```python
from build123d import *

# Parameters (mm, degrees)
SKETCH044_W             = 574.323184
SKETCH044_H             = 18
PAD022_DEPTH            = 8
SKETCH049_R             = 2
POCKET031_DEPTH         = 8.001
CHAMFER017_SIZE         = 3
SKETCH050_W             = 25
SKETCH050_H             = 18
POCKET032_DEPTH         = 5.5
SKETCH070_R             = 2
POCKET045_DEPTH         = 8.001
CHAMFER029_SIZE         = 3
BODY016_PLACEMENT_ANGLE = 180


with BuildPart() as part:
    # Sketch044 → Pad022 (new body)
    with BuildSketch(Plane.XY):
        with Locations((57.838408, -99)):
            Rectangle(SKETCH044_W, SKETCH044_H)
    extrude(amount=PAD022_DEPTH)

    # Sketch049 (on Face6 of Pad022) → Pocket031 (cut, through all)
    with BuildSketch(Plane.XY.offset(8)):
        with Locations((316, -99)):
            Circle(SKETCH049_R)
        with Locations((336, -99)):
            Circle(SKETCH049_R)
    extrude(amount=-POCKET031_DEPTH, mode=Mode.SUBTRACT)

    # Chamfer017
    chamfer017_edges = [part.edges().sort_by_distance(p)[0] for p in [
        (334, -99, 8),
        (314, -99, 8),
    ]]
    chamfer(chamfer017_edges, length=CHAMFER017_SIZE)

    # Sketch050 (on Face9 of Chamfer017) → Pocket032 (cut)
    with BuildSketch(Plane(origin=(0, 0, 0), x_dir=(1, 0, 0), z_dir=(0, 0, -1))):
        with Locations((-183.823184, 99)):
            Rectangle(SKETCH050_W, SKETCH050_H)
        with Locations((-93.823184, 99)):
            Rectangle(SKETCH050_W, SKETCH050_H)
        with Locations((-3.823184, 99)):
            Rectangle(SKETCH050_W, SKETCH050_H)
        with Locations((86.176816, 99)):
            Rectangle(SKETCH050_W, SKETCH050_H)
    extrude(amount=-POCKET032_DEPTH, mode=Mode.SUBTRACT)

    # Sketch070 (on Face1 of Pocket032) → Pocket045 (cut, through all)
    with BuildSketch(Plane.XY.offset(8)):
        with Locations((-48.823184, -99)):
            Circle(SKETCH070_R)
    extrude(amount=-POCKET045_DEPTH, mode=Mode.SUBTRACT)

    # Chamfer029
    chamfer029_edges = [part.edges().sort_by_distance(p)[0] for p in [
        (-50.823184, -99, 0),
    ]]
    chamfer(chamfer029_edges, length=CHAMFER029_SIZE)


with BuildPart() as part_1:
    # Body016 placement: moved
    add(part.part.moved(Location((0, 0, 15.5))).rotate(Axis((0, 0, 15.5), (1, 0, 0)), BODY016_PLACEMENT_ANGLE))


solid = part_1.part
```
Work out the finished part from the listing and answer in its coordinate system (mm). A direction names the side the tool comes from. Give positions to 0.01 mm unless a question says otherwise; leave off trailing zeros. One line per item, written item: value. Start each with the question number.
1. Which of the six approach directions +Z, -Z, +X, -X, +Y, -Y give full straight-line access (tool end or side, diameter ignored) to faces 3 (the face through (54, 99, 7.5)), 4 (the face through (-4, 99, 10))?
2. Each of these flat-tipped pins is pushed along its axis until it touches: pin 1 Ø5.5 at (x, y) = (83.5, 95) entering from +Z; pin 2 Ø6.5 at (x, y) = (336, 99) entering from -Z; pin 3 Ø4.5 at (x, y) = (316, 99) entering from -Z. Where does it stop, or does it pass through?
3. Consider line 1 (X direction, y = 95, z = 11.5); line 2 (Y direction, x = 316, z = 14.2); line 3 (Z direction, x = 7.5, y = 104.5). Determine where each line is inside the solid, lowest interval first.
4. For a pull along Y with two mould halves and no side action, classify faces 1 (the face through (313.856, 98.906, 10.354)), 2 (the face through (220, 99, 15.5)) as released by +Y, released by -Y, zero draft, split by the parting line, or undercut.
Filled sheet:
1. face 3: -Z, +X, -X, +Y, -Y
1. face 4: +Z, +Y, -Y
2. pin 1: z = 10
2. pin 2: z = 9.25
2. pin 3: z = 10.25
3. line 1: -229.32 to -196.32, -171.32 to -106.32, -81.32 to -16.32, 8.68 to 73.68, 98.68 to 345
3. line 2: 90 to 97, 101 to 108
3. line 3: 7.5 to 10
4. face 1: undercut
4. face 2: zero draft
